The model under review builds one solid part; all positions refer to its coordinate system, in mm. A direction names the side the tool comes from. Give positions to 0.01 mm unless a question says otherwise; leave off trailing zeros. Loops run counter-clockwise (first coordinate to the right, second up) from the corner with the lowest first, then second, coordinate; pieces in that order, holes last. Notation, with made-up numbers: (54.5, 52.25) - (108.5, 52.25) arc R22 cw to (108.5, 87.25) - close; hole circle Ø7 at (30, 10.5). An arc over 180 degrees is marked (long way). Answer as a JSON object with one key per item and string values.
from build123d import *

# Parameters (mm, degrees)
SKETCH1_R           = 3
BOSS_EXTRUDE1_DEPTH = 4
CUT_EXTRUDE3_DEPTH  = 82.313525364
CUT_EXTRUDE2_DEPTH  = 1.25
SKETCH6_R           = 4.25
SKETCH6_R_2         = 3
BOSS_EXTRUDE2_DEPTH = 1.25
SKETCH7_R           = 4.25
CUT_EXTRUDE4_DEPTH  = 1.2


with BuildPart() as part:
    # Sketch1 → Boss-Extrude1 (new, symmetric)
    with BuildSketch(Plane.XY):
        with BuildLine():
            Line((0, -6.35), (0, 0))
            Line((0, 0), (49.523071285, 6.889514534))
            ThreePointArc((49.523071285, 6.889514534), (55.424924624, 0.340905899), (63.899469217, -2.087723723))
            Line((63.899469217, -2.087723723), (73, -2.087723723))
            ThreePointArc((73, -2.087723723), (79.5, -8.587723723), (73, -15.087723723))
            Line((73, -15.087723723), (22.2, -15.087723723))
            Line((22.2, -15.087723723), (0, -6.35))
        make_face()
        with Locations((73, -8.587723723)):
            Circle(SKETCH1_R, mode=Mode.SUBTRACT)
        with Locations((22.2, -8.587723723)):
            Circle(SKETCH1_R, mode=Mode.SUBTRACT)
    extrude(amount=BOSS_EXTRUDE1_DEPTH, both=True)

    # Sketch5 → Cut-Extrude3 (cut, through all)
    with BuildSketch(Plane.XY.offset(4)):
        Polygon((4.952307128, 0.688951453), (0, 0), (2.675036718, -1.0851322), align=None)
        Polygon((49.523071285, 6.889514534), (44.570764156, 6.200563081), (47.245800874, 5.115430881), align=None)
        Polygon((44.570764156, 6.200563081), (39.618457028, 5.511611627), (42.293493746, 4.426479427), align=None)
        Polygon((39.618457028, 5.511611627), (34.666149899, 4.822660174), (37.341186617, 3.737527974), align=None)
        Polygon((34.666149899, 4.822660174), (29.713842771, 4.133708721), (32.388879489, 3.04857652), align=None)
        Polygon((29.713842771, 4.133708721), (24.761535642, 3.444757267), (27.43657236, 2.359625067), align=None)
        Polygon((24.761535642, 3.444757267), (19.809228514, 2.755805814), (22.484265232, 1.670673614), align=None)
        Polygon((19.809228514, 2.755805814), (14.856921385, 2.06685436), (17.531958103, 0.98172216), align=None)
        Polygon((14.856921385, 2.06685436), (9.904614257, 1.377902907), (12.579650975, 0.292770707), align=None)
        Polygon((9.904614257, 1.377902907), (4.952307128, 0.688951453), (7.627343846, -0.396180747), align=None)
    extrude(amount=-CUT_EXTRUDE3_DEPTH, mode=Mode.SUBTRACT)

    # Sketch4 → Cut-Extrude2 (cut)
    with BuildSketch(Plane.XY.offset(4)):
        with BuildLine():
            Line((22.579425451, -13.087723723), (73, -13.087723723))
            ThreePointArc((73, -13.087723723), (77.5, -8.587723723), (73, -4.087723723))
            Line((73, -4.087723723), (63.899469217, -4.087723723))
            ThreePointArc((63.899469217, -4.087723723), (55.420413641, -1.965557849), (48.940687218, 3.900541107))
            Line((48.940687218, 3.900541107), (47.56401392, 2.828058198))
            Line((47.56401392, 2.828058198), (44.888977202, 3.913190398))
            Line((44.888977202, 3.913190398), (42.611706791, 2.139106744))
            Line((42.611706791, 2.139106744), (39.936670074, 3.224238944))
            Line((39.936670074, 3.224238944), (37.659399663, 1.450155291))
            Line((37.659399663, 1.450155291), (34.984362945, 2.535287491))
            Line((34.984362945, 2.535287491), (32.707092534, 0.761203837))
            Line((32.707092534, 0.761203837), (30.032055817, 1.846336038))
            Line((30.032055817, 1.846336038), (27.754785406, 0.072252384))
            Line((27.754785406, 0.072252384), (25.079748688, 1.157384584))
            Line((25.079748688, 1.157384584), (22.802478277, -0.616699069))
            Line((22.802478277, -0.616699069), (20.12744156, 0.468433131))
            Line((20.12744156, 0.468433131), (17.850171149, -1.305650523))
            Line((17.850171149, -1.305650523), (15.175134431, -0.220518323))
            Line((15.175134431, -0.220518323), (12.89786402, -1.994601976))
            Line((12.89786402, -1.994601976), (10.222827303, -0.909469776))
            Line((10.222827303, -0.909469776), (7.945556892, -2.68355343))
            Line((7.945556892, -2.68355343), (5.270520174, -1.59842123))
            Line((5.270520174, -1.59842123), (2.993249763, -3.372504883))
            Line((2.993249763, -3.372504883), (2, -2.969591796))
            Line((2, -2.969591796), (2, -4.987843814))
            Line((2, -4.987843814), (22.579425451, -13.087723723))
        make_face()
    extrude(amount=-CUT_EXTRUDE2_DEPTH, mode=Mode.SUBTRACT)

    # Sketch6 → Boss-Extrude2 (add)
    # profile 1 of 2: a face of its own
    with BuildSketch(Plane.XY.offset(2.75)):
        with Locations((22.2, -8.587723723)):
            Circle(SKETCH6_R)
        with Locations((22.2, -8.587723723)):
            Circle(SKETCH6_R_2, mode=Mode.SUBTRACT)
    # profile 2 of 2: a face of its own
    with BuildSketch(Plane.XY.offset(2.75)):
        with Locations((73, -8.587723723)):
            Circle(SKETCH6_R)
        with Locations((73, -8.587723723)):
            Circle(SKETCH6_R_2, mode=Mode.SUBTRACT)
    extrude(amount=BOSS_EXTRUDE2_DEPTH)

    # Sketch7 → Cut-Extrude4 (cut)
    with BuildSketch(Plane(origin=(0, 0, -4), x_dir=(-1, 0, 0), z_dir=(0, 0, -1))):
        with BuildLine():
            Line((-20.12744156, 0.468433131), (-22.802478277, -0.616699069))
            Line((-22.802478277, -0.616699069), (-25.079748688, 1.157384584))
            Line((-25.079748688, 1.157384584), (-27.754785406, 0.072252384))
            Line((-27.754785406, 0.072252384), (-30.032055817, 1.846336038))
            Line((-30.032055817, 1.846336038), (-32.707092534, 0.761203837))
            Line((-32.707092534, 0.761203837), (-34.984362945, 2.535287491))
            Line((-34.984362945, 2.535287491), (-37.659399663, 1.450155291))
            Line((-37.659399663, 1.450155291), (-39.936670074, 3.224238944))
            Line((-39.936670074, 3.224238944), (-42.611706791, 2.139106744))
            Line((-42.611706791, 2.139106744), (-44.888977202, 3.913190398))
            Line((-44.888977202, 3.913190398), (-47.56401392, 2.828058198))
            Line((-47.56401392, 2.828058198), (-48.940687218, 3.900541107))
            ThreePointArc((-48.940687218, 3.900541107), (-55.420413641, -1.965557849), (-63.899469217, -4.087723723))
            Line((-63.899469217, -4.087723723), (-73, -4.087723723))
            ThreePointArc((-73, -4.087723723), (-77.5, -8.587723723), (-73, -13.087723723))
            Line((-73, -13.087723723), (-22.579425451, -13.087723723))
            Line((-22.579425451, -13.087723723), (-21.920947479, -12.828552615))
            ThreePointArc((-21.920947479, -12.828552615), (-23.756536974, -4.633018595), (-19.513668259, -11.881068798))
            Line((-19.513668259, -11.881068798), (-2, -4.987843814))
            Line((-2, -4.987843814), (-2, -2.969591796))
            Line((-2, -2.969591796), (-2.993249763, -3.372504883))
            Line((-2.993249763, -3.372504883), (-5.270520174, -1.59842123))
            Line((-5.270520174, -1.59842123), (-7.945556892, -2.68355343))
            Line((-7.945556892, -2.68355343), (-10.222827303, -0.909469776))
            Line((-10.222827303, -0.909469776), (-12.89786402, -1.994601976))
            Line((-12.89786402, -1.994601976), (-15.175134431, -0.220518323))
            Line((-15.175134431, -0.220518323), (-17.850171149, -1.305650523))
            Line((-17.850171149, -1.305650523), (-20.12744156, 0.468433131))
        make_face()
        with Locations(Location((-73, -8.587723723, 0), (0, 0, 180))):
            Circle(SKETCH7_R, mode=Mode.SUBTRACT)
    extrude(amount=-CUT_EXTRUDE4_DEPTH, mode=Mode.SUBTRACT)


solid = part.part
Q1. Consider section A-A, the plane z = 1.5. State the section outline as (x, y) points, plus the area to 3 significant figures.
Results:
{"outline": "(0, -6.35) - (22.2, -15.09) - (73, -15.09) arc R6.5 ccw to (73, -2.09) - (63.9, -2.09) arc R16 cw to (49.52, 6.89) - (47.25, 5.12) - (44.57, 6.2) - (42.29, 4.43) - (39.62, 5.51) - (37.34, 3.74) - (34.67, 4.82) - (32.39, 3.05) - (29.71, 4.13) - (27.44, 2.36) - (24.76, 3.44) - (22.48, 1.67) - (19.81, 2.76) - (17.53, 0.98) - (14.86, 2.07) - (12.58, 0.29) - (9.9, 1.38) - (7.63, -0.4) - (4.95, 0.69) - (2.68, -1.09) - (0, 0) - close; hole circle Ø6 at (22.2, -8.59); hole circle Ø6 at (73, -8.59)", "area": "1,140 mm^2"}
Q2. The part is to be moulded in two halves that separate along Y. For faces 6 (the face through (43.77, 3.04, 3.38)), 7 (the face through (48, -15.088, 0)), 8 (the face through (48.37, 5.99, 0.06)), say which applies: +Y half, -Y half, draft (parallel to the pull), parting line (faces both ways), or undercut.
Results:
{"face 6": "undercut", "face 7": "-Y half", "face 8": "+Y half"}
Q3. For faces 1 (the face through (33.83, 1.636, -3.408)), 2 (the face through (35.98, 4.29, 0.06)), 3 (the face through (68, -2.088, 0)), 4 (the face through (76, -10, 4)), 5 (the face through (11.58, -1.46, 3.38)), list the 3-axis set-ups (+Z, -Z, +X, -X, +Y, -Y) from which the entire face can be reached by the end or side of a thin tool; tool diameter is ignored.
Results:
{"face 1": "-Z", "face 2": "+Z, -Z, +Y", "face 3": "+Z, -Z, +X, +Y", "face 4": "+Z, +X, -X, +Y, -Y", "face 5": "+Z"}
Q4. Clearance check with flat-ended pins moving along their axes: pin 1 Ø1.3 at (y, z) = (-4.5, -3.5) entering from +X; pin 2 Ø1 at (x, z) = (39, 3.5) entering from +Y; pin 3 Ø1 at (x, z) = (62, 2.5) entering from +Y; pin 4 Ø3.5 at (x, y) = (73, -8.59) entering from +Z. State where each tip first meets the part, or that it passes through.
Results:
{"pin 1": "stops at x = 78.52", "pin 2": "stops at y = 5.42", "pin 3": "stops at y = -1.91", "pin 4": "passes through"}
Q5. To check wall thickness, follow probe 1 along X at (y, z) = (2, 1); probe 2 along Y at (x, z) = (73, -0.25); probe 3 along Z at (x, y) = (26.5, -10). State the ranges of each line that lie inside material, in increasing order. Write a range as [from, to].
Results:
{"probe 1": "x = [14.77, 15.02], [18.84, 21.67], [22.91, 53.22]", "probe 2": "y = [-15.09, -11.59], [-5.59, -2.09]", "probe 3": "z = [-2.8, 2.75]"}
